Autodesk Inventor part; units mm, degrees
ref_plane "YZ Plane" through (0, 0, 0) normal (1, 0, 0) x (0, 1, 0)
ref_plane "XZ Plane" through (0, 0, 0) normal (0, 1, 0) x (-1, 0, 0)
ref_plane "XY Plane" through (0, 0, 0) normal (0, 0, 1) x (1, 0, 0)
sketch "Sketch1" plane through (0, 0, 0) normal (1, 0, 0) x (0, 1, 0)
  circle A0 centre (0, 0) radius 4
  arc A1 (-2.4231, 3.7919) -> (2.4231, 3.7919) centre (0, 0) ccw
  line L0 (-1.5, 11.2085) -> (-1.5, 5.4772)
  line L1 (1.5, 5.4772) -> (1.5, 11.2085)
  arc A2 (1.5, 5.4772) -> (2.4231, 3.7919) centre (3.5, 5.4772) ccw
  arc A3 (-2.4231, 3.7919) -> (-1.5, 5.4772) centre (-3.5, 5.4772) ccw
  line L2 (0.5, 12.2085) -> (-0.5, 12.2085)
  arc A4 (1.5, 11.2085) -> (0.5, 12.2085) centre (0.5, 11.2085) ccw
  arc A5 (-0.5, 12.2085) -> (-1.5, 11.2085) centre (-0.5, 11.2085) ccw
  point P0 (-1.5, 4.2426)
  point P1 (1.5, 4.2426)
  dimension "d0" = 8
  dimension "d1" = 9
  dimension "d4" = 2
  dimension "d8" = 1
extrude "Extrusion1" add sketch "Sketch1" along normal blind 2
properties part number "_3DPrint"
Geometry: final body of the model. Coordinates: model frame, mm. A direction names the side the tool comes from. Coordinates: 2 decimals unless noted, no trailing zeros. Order: outer loops, then holes, each group sorted by start corner. A loop starts at its lowest first (then second) coordinate and runs counter-clockwise, first axis right, second up. Notation, with made-up numbers: (18.5, 13) -> (22.5, 13) arc R16 ccw to (22.5, 37) -> close; hole circle Ø4 at (60, 75.5). An arc over 180 degrees is marked (long way). Write each question's results on one line, items separated by ' | '. Start each with the question number.
1) First-contact query: pin 1 (0.6 mm diameter, centred on x = 1, z = 8.5, fed in from +Y). Flat tip, straight axial feed; report the tip coordinate or a pass-through.
2) Cut plane C-C, the plane x = 0.55. Output: boundary loops of the cut face in (y, z).
3) Mould query, pull axis Y, two halves, no side actions, for faces 1 (the cylindrical face through (0.986, -0.867, 3.905)), 2 (the cylindrical face through (0.99, -1.21, 11.91)), 3 (the flat face through (1, 1.5, 8)). Classes: released by +Y, released by -Y, zero draft, split by the parting line, or undercut.
4) Cut plane A-A, the plane y = 0. Output: boundary loops of the cut face in (x, z), and give its area (3 significant figures).
5) Set-up query: faces 4 (the flat face through (0, 0, 5)), 5 (the flat face through (1, -1.5, 8)). Return all of +Z, -Z, +X, -X, +Y, -Y with unobstructed straight access to the full face (end or side cutting, diameter ignored); none if empty.
6) Cut plane B-B, the plane z = 0. Output: boundary loops of the cut face in (x, y), and give its area (3 significant figures).
7) Cut plane D-D, the plane z = 11. Output: boundary loops of the cut face in (x, y), and give its area (3 significant figures).
8) Material intervals for line 1 along Y through (x, z) = (1.05, -2.5); line 2 along Z through (x, y) = (1.1, 1.75); line 3 along Z through (x, y) = (0.25, -3.25), sorted ascending.
Checks:
1) pin 1: y = 1.5
2) outline: (-2.42, 3.79) arc R4.5 ccw (long way) to (2.42, 3.79) arc R2 cw to (1.5, 5.48) -> (1.5, 11.21) arc R1 ccw to (0.5, 12.21) -> (-0.5, 12.21) arc R1 ccw to (-1.5, 11.21) -> (-1.5, 5.48) arc R2 cw to start; hole circle Ø8 at (0, 0)
3) face 1: undercut | face 2: released by -Y | face 3: released by +Y
4) outline: (0, -4.5) -> (2, -4.5) -> (2, -4) -> (0, -4) -> close; (0, 4) -> (2, 4) -> (2, 12.21) -> (0, 12.21) -> close | area: 17.4 mm^2
5) face 4: +Z, -Z, -X, +Y, -Y | face 5: +Z, +X, -X, -Y
6) outline: (0, -4.5) -> (2, -4.5) -> (2, -4) -> (0, -4) -> close; (0, 4) -> (2, 4) -> (2, 4.5) -> (0, 4.5) -> close | area: 2.00 mm^2
7) outline: (0, -1.5) -> (2, -1.5) -> (2, 1.5) -> (0, 1.5) -> close | area: 6.00 mm^2
8) line 1: -3.74 to -3.12, 3.12 to 3.74 | line 2: -4.15 to -3.6, 3.6 to 4.51 | line 3: -3.11 to -2.33, 2.33 to 3.11
